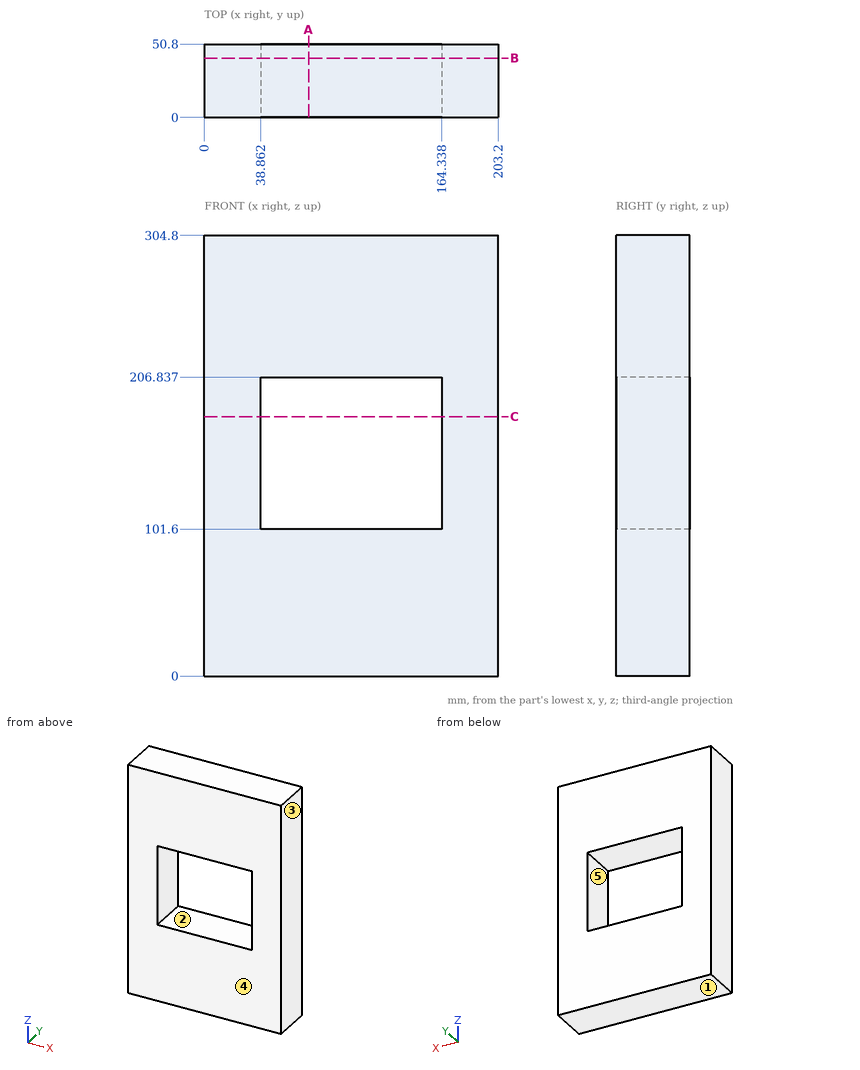
Drawing for the job (mm, zero at the part's lowest x, y, z). A direction names the side the tool comes from. Round coordinates to 2 decimals unless told otherwise and drop trailing zeros. Write each loop counter-clockwise with the first axis right and the second up, starting at its lowest first coordinate (ties: lowest second). Pieces come first, ordered by that corner, then holes. Notation, with made-up numbers: M -5.75,40 L 9.25,40 A31 cw 9.25,77 Z; hole C 33.25,12.25 d1. An arc over 180 degrees is marked long. Answer in a Markdown table with one row per item.
1. Saw through at A-A (x = 72). List the corners of the cut face in (y, z).
Geometry check:
| item | result |
|---|---|
| outline | M 0,0 L 50.8,0 L 50.8,101.6 L 0,101.6 Z; M 0,206.84 L 50.8,206.84 L 50.8,304.8 L 0,304.8 Z |
2. Saw through at B-B (y = 41). List the corners of the cut face in (x, z).
Geometry check:
| item | result |
|---|---|
| outline | M 0,0 L 203.2,0 L 203.2,304.8 L 0,304.8 Z; hole M 38.86,101.6 L 164.34,101.6 L 164.34,206.84 L 38.86,206.84 Z |
3. Which spindle directions (+Z, -Z, +X, -X, +Y, -Y) get a long thin tool onto all of the face, cutting with end or side? Do the marked faces 4 and 5. Say none if no direction does.
Geometry check:
| item | result |
|---|---|
| face 4 | +Z, -Z, +X, -X, -Y |
| face 5 | +Y, -Y |
4. Probe L1, parallel to Z at x = 107, y = 26.5; L2, parallel to X at y = 44.5, z = 109.5. List the from-to ranges inside material, lowest first. Write a range as [from, to].
Geometry check:
| item | result |
|---|---|
| L1 | [0, 101.6], [206.84, 304.8] |
| L2 | [0, 38.86], [164.34, 203.2] |
5. Flat gauge pin, fed straight in: P1, Ø6, axis at x = 159, z = 161.5, coming from the -Y side. Where does the tip first touch, or does it go through?
Geometry check:
| item | result |
|---|---|
| P1 | through |
6. Mould opens along X. For the marked faces 1, 2 and 3 say: +X half, -X half, draft (parallel to the pull), parting line (faces both ways), or undercut.
Geometry check:
| item | result |
|---|---|
| face 1 | draft |
| face 2 | undercut |
| face 3 | +X half |
7. Saw through at C-C (z = 179.5). List the corners of the cut face in (x, y), and give its area (3 significant figures).
Geometry check:
| item | result |
|---|---|
| outline | M 0,0 L 38.86,0 L 38.86,50.8 L 0,50.8 Z; M 164.34,0 L 203.2,0 L 203.2,50.8 L 164.34,50.8 Z |
| area | 3,950 mm2 |
